from build123d import *

# Parameters (mm, degrees)
SKETCH4_R           = 1.901825
BOSS_EXTRUDE1_DEPTH = 12.7
SKETCH5_OUTSIDE_W   = 75.8
SKETCH5_OUTSIDE_H   = 76.538
SKETCH5_OUTSIDE_R   = 2.2621875
CUT_EXTRUDE1_DEPTH  = 18.837312762
CUT_EXTRUDE1_DRAFT  = -60
SKETCH6_OUTSIDE_W   = 59.772
SKETCH6_OUTSIDE_H   = 60.51
SKETCH6_OUTSIDE_R   = 2.2621875
CUT_EXTRUDE2_DEPTH  = 14.210632851
CUT_EXTRUDE2_DRAFT  = -60
FILLET1_R           = 0.47625


with BuildPart() as part:
    # Sketch3 → Revolve1 (revolve)
    with BuildSketch(Plane(origin=(0, 0, 0), x_dir=(0, 0, -1), z_dir=(1, 0, 0))):
        with BuildLine():
            Line((-6.35, 1.26365), (-6.35, 0))
            Line((-6.35, 0), (4.7625, 0))
            Line((4.7625, 0), (4.7625, 1.26365))
            Line((4.7625, 1.26365), (4.60375, 1.4224))
            Line((4.60375, 1.4224), (0.809625, 1.4224))
            Line((0.809625, 1.4224), (0.5715, 1.009955401))
            Line((0.5715, 1.009955401), (0.15875, 1.009955401))
            ThreePointArc((0.15875, 1.009955401), (0.046496798, 1.0564522), (0, 1.168705401))
            Line((0, 1.168705401), (0, 2.38125))
            Line((0, 2.38125), (-12.7, 2.38125))
            Line((-12.7, 2.38125), (-12.7, 1.58115))
            Line((-12.7, 1.58115), (-12.54125, 1.4224))
            Line((-12.54125, 1.4224), (-6.50875, 1.4224))
            Line((-6.50875, 1.4224), (-6.35, 1.26365))
        make_face()
    revolve(axis=Axis((0, 0, -4.7625), (0, 0, 1)))

    # Sketch4 → Boss-Extrude1 (add)
    with BuildSketch(Plane.XY.offset(12.7)):
        Polygon((-2.38125, 1.374815329), (-2.38125, -1.374815329), (0, -2.749630657), (2.38125, -1.374815329), (2.38125, 1.374815329), (0, 2.749630657), align=None)
        Circle(SKETCH4_R, mode=Mode.SUBTRACT)
    extrude(amount=-BOSS_EXTRUDE1_DEPTH)


with BuildPart() as cut_extrude1_tool:
    # Sketch5 outside → Cut-Extrude1 (with draft: the straight prism first)
    with BuildSketch(Plane.XY.offset(12.7)):
        Rectangle(SKETCH5_OUTSIDE_W, SKETCH5_OUTSIDE_H)
        Circle(SKETCH5_OUTSIDE_R, mode=Mode.SUBTRACT)
    extrude(amount=-CUT_EXTRUDE1_DEPTH)
    # Cut-Extrude1: the draft: its side faces are tilted about the plane it starts from
    cut_extrude1_sides = [cut_extrude1_tool.faces().sort_by_distance(p)[0] for p in [
        (0, -38.269, 3.281343619),
        (37.9, 0, 3.281343619),
        (0, 38.269, 3.281343619),
        (-37.9, 0, 3.281343619),
        (-2.2621875, 0, 3.281343619),
    ]]
    draft(cut_extrude1_sides, Plane.XY.offset(12.7), CUT_EXTRUDE1_DRAFT)


with BuildPart() as part_1:
    add(part.part)

    # Cut-Extrude1: cut by cut_extrude1_tool
    add(cut_extrude1_tool.part, mode=Mode.SUBTRACT)


with BuildPart() as cut_extrude2_tool:
    # Sketch6 outside → Cut-Extrude2 (with draft: the straight prism first)
    with BuildSketch(Plane(origin=(0, 0, 0), x_dir=(-1, 0, 0), z_dir=(0, 0, -1))):
        Rectangle(SKETCH6_OUTSIDE_W, SKETCH6_OUTSIDE_H)
        Circle(SKETCH6_OUTSIDE_R, mode=Mode.SUBTRACT)
    extrude(amount=-CUT_EXTRUDE2_DEPTH)
    # Cut-Extrude2: the draft: its side faces are tilted about the plane it starts from
    cut_extrude2_sides = [cut_extrude2_tool.faces().sort_by_distance(p)[0] for p in [
        (0, -30.255, 7.105316425),
        (-29.886, 0, 7.105316425),
        (0, 30.255, 7.105316425),
        (29.886, 0, 7.105316425),
        (2.2621875, 0, 7.105316425),
    ]]
    draft(cut_extrude2_sides, Plane(origin=(0, 0, 0), x_dir=(-1, 0, 0), z_dir=(0, 0, -1)), CUT_EXTRUDE2_DRAFT)


with BuildPart() as part_2:
    add(part_1.part)

    # Cut-Extrude2: cut by cut_extrude2_tool
    add(cut_extrude2_tool.part, mode=Mode.SUBTRACT)

    # Fillet1
    fillet1_edges = [part_2.edges().sort_by_distance(p)[0] for p in [
        (0, 2.749630657, 6.35),
        (-2.38125, -1.374815329, 6.35),
        (0, -2.749630657, 6.35),
        (2.38125, -1.374815329, 6.35),
        (2.38125, 1.374815329, 6.35),
        (-2.38125, 1.374815329, 6.35),
    ]]
    fillet(fillet1_edges, radius=FILLET1_R)


solid = part_2.part
Geometry: final body of the model. Coordinates: model frame, mm. A direction names the side the tool comes from. Coordinates: 2 decimals unless noted, no trailing zeros. Order: outer loops, then holes, each group sorted by start corner. A loop starts at its lowest first (then second) coordinate and runs counter-clockwise, first axis right, second up.
(1) Section query A-A (x = 0). Return the cut outline in (y, z), plus the area to 3 significant figures.
(2) Section query B-B (y = 0). Return the cut outline in (x, z).
(3) Access query for faces 1 (the face through (0, 0, 6.35)), 2 (the face through (0.615, -0.801, -0.362)), 3 (the face through (-1.18, 2.07, 6.44)). Directions: +Z, -Z, +X, -X, +Y, -Y. A direction counts if a zero-diameter tool reaches every point of the face in a straight line with its end or side. Return the directions, or none.
(4) First-contact query: pin 1 (1.5 mm diameter, centred on x = -1.5, z = 5, fed in from +Y); pin 2 (1 mm diameter, centred on x = 0.5, z = 2.5, fed in from +Y). Flat tips, straight axial feed; report the tip coordinate or a pass-through.
(5) Section query C-C (z = 3.25). Return the cut outline in (x, y) (1 decimal), plus the area to 3 significant figures.
(6) Draft query along Y for faces 4 (the face through (1.39, -0.31, -2.68)), 5 (the face through (1, -1, 0)), 6 (the face through (1.39, -0.31, 9.48)). Return one class per face: pulls with the +Y half, pulls with the -Y half, needs draft (parallel to the pull), parting line crosses it, or undercut.
(7) Section query D-D (z = -3.25). Return the cut outline in (x, y), plus the area to 3 significant figures.
(8) Material intervals for probe 1 along Y at (x, z) = (0, 8.25); probe 2 along X at (y, z) = (0, 10); probe 3 along Z at (x, y) = (-0.05, 0.3), sorted ascending.
Solution:
1. outline: (-2.68, 0.24) - (-2.26, 0) - (-1.17, 0) arc R0.16 cw to (-1.01, -0.16) - (-1.01, -0.57) - (-1.42, -0.81) - (-1.42, -4.6) - (-1.26, -4.76) - (1.26, -4.76) - (1.42, -4.6) - (1.42, -0.81) - (1.01, -0.57) - (1.01, -0.16) arc R0.16 cw to (1.17, 0) - (2.26, 0) - (2.68, 0.24) - (2.68, 12.46) - (2.26, 12.7) - (1.58, 12.7) - (1.42, 12.54) - (1.42, 6.51) - (1.26, 6.35) - (-1.26, 6.35) - (-1.42, 6.51) - (-1.42, 12.54) - (-1.58, 12.7) - (-2.26, 12.7) - (-2.68, 12.46) - close
1. area: 62.7 mm2
2. outline: (-2.38, 0.07) - (-2.26, 0) - (-1.17, 0) arc R0.16 cw to (-1.01, -0.16) - (-1.01, -0.57) - (-1.42, -0.81) - (-1.42, -4.6) - (-1.26, -4.76) - (1.26, -4.76) - (1.42, -4.6) - (1.42, -0.81) - (1.01, -0.57) - (1.01, -0.16) arc R0.16 cw to (1.17, 0) - (2.26, 0) - (2.38, 0.07) - (2.38, 12.63) - (2.26, 12.7) - (1.58, 12.7) - (1.42, 12.54) - (1.42, 6.51) - (1.26, 6.35) - (-1.26, 6.35) - (-1.42, 6.51) - (-1.42, 12.54) - (-1.58, 12.7) - (-2.26, 12.7) - (-2.38, 12.63) - close
3. face 1: +Z
3. face 2: none
3. face 3: +Z, -Z, -X, +Y
4. pin 1: stops at y = 2.32
4. pin 2: stops at y = 2.68
5. outline: (-2.4, -1.1) arc R0.5 ccw to (-2.1, -1.5) - (-0.2, -2.6) arc R0.5 ccw to (0.2, -2.6) - (2.1, -1.5) arc R0.5 ccw to (2.4, -1.1) - (2.4, 1.1) arc R0.5 ccw to (2.1, 1.5) - (0.2, 2.6) arc R0.5 ccw to (-0.2, 2.6) - (-2.1, 1.5) arc R0.5 ccw to (-2.4, 1.1) - close
5. area: 19.6 mm2
6. face 4: parting line crosses it
6. face 5: needs draft
6. face 6: undercut
7. outline: circle Ø2.84 at (0, 0)
7. area: 6.36 mm2
8. probe 1: y = -2.68 to -1.42, 1.42 to 2.68
8. probe 2: x = -2.38 to -1.42, 1.42 to 2.38
8. probe 3: z = -4.76 to 6.35
